The listing builds one solid part. Answer for the finished solid, in the listing's coordinates (mm). Face numbers are marked on the shaded views. A direction names the side the tool comes from. Round coordinates to 2 decimals unless told otherwise and drop trailing zeros. Write each loop counter-clockwise with the first axis right and the second up, starting at its lowest first coordinate (ties: lowest second). Pieces come first, ordered by that corner, then holes. Notation, with made-up numbers: (80.5, -29) - (112.5, -29) arc R11 cw to (112.5, -15) - close; hole circle Ø1 at (55.5, 72). An arc over 180 degrees is marked (long way). Use a Markdown table: item, result. Add a question column.
1) A cutting plane is placed at A-A (y = 11.25). Give the vertices of the cut face in (x, z) (3 decimals).
2) A cutting plane is placed at B-B (x = -10.5). Give the vertices of the cut face in (y, z), then the cut area to 3 significant figures.
3) A cutting plane is placed at D-D (z = 4.5). Give the vertices of the cut face in (x, y).
4) A tool of negligible diameter and unlimited length cuts with its end or side. For the marked faces 5, 6, 7 and 8, from which of +Z, -Z, +X, -X, +Y, -Y can it reach the whole face along a straight path? Write none if from no direction.
5) Determine the mould class of the marked faces 1, 2, 3 and 4 for opening direction X: +X half, -X half, draft (parallel to the pull), parting line (faces both ways), or undercut.
6) Each of these flat-tipped pins is pushed along its axis until it touches: P1, Ø2, axis at x = -22.5, z = -3.5, coming from the +Y side; P2, Ø0.6, axis at y = 2, z = 6, coming from the +X side; P3, Ø0.7, axis at y = 0.5, z = 5.5, coming from the +X side (3 decimals); P4, Ø3, axis at x = -5.5, z = 3.5, coming from the +Y side. Where does it stop, or does it pass through?
7) A cutting plane is placed at C-C (z = -4.5). Give the vertices of the cut face in (x, y) (3 decimals).
8) Find the intervals of material crossed by probe 1 along X at (y, z) = (1.1, 3.1) (3 decimals); probe 2 along X at (y, z) = (2.1, 3.1) (3 decimals); probe 3 along X at (y, z) = (9, -2.5) (3 decimals), in increasing order. Write a range as from..to.
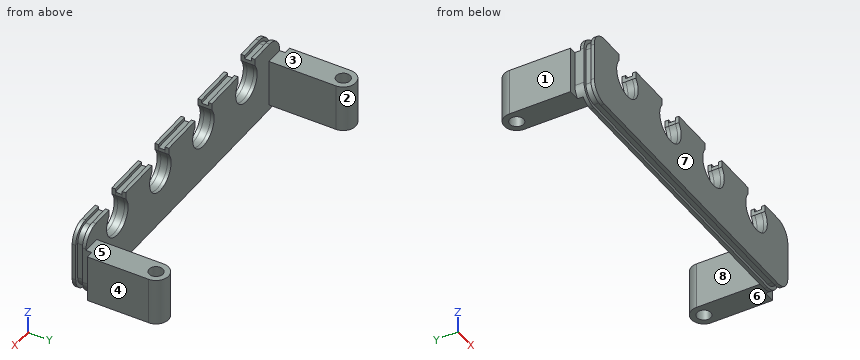
```python
from build123d import *
from build123d import SkipClean  # not in build123d's __all__

# Parameters (mm, degrees)
F1_DEPTH = 0.64
F3_DEPTH = 1.21
F5_DEPTH = 0.64
F7_R     = 1.25
F8_DEPTH = 8.5
F9_DEPTH = 1


# Not quite as in the source:
# - after a boolean that leaves OpenCascade's solid faulty, fix() repairs it


with BuildPart() as f1:
    # F0 (on Front) → F1 (new body)
    with BuildSketch(Plane.XZ):
        with BuildLine():
            ThreePointArc((-29.225, -3.35), (-28.3463203436, -5.4713203436), (-26.225, -6.35))
            Line((-26.225, -6.35), (26.225, -6.35))
            ThreePointArc((26.225, -6.35), (28.3463203436, -5.4713203436), (29.225, -3.35))
            Line((29.225, -3.35), (29.225, 3.35))
            ThreePointArc((29.225, 3.35), (28.3463203436, 5.4713203436), (26.225, 6.35))
            Line((26.225, 6.35), (22.325, 6.35))
            Line((22.325, 6.35), (22.325, 5.114944168))
            ThreePointArc((22.325, 5.114944168), (19.775, -0.15), (17.225, 5.114944168))
            Line((17.225, 5.114944168), (17.225, 6.35))
            Line((17.225, 6.35), (9.325, 6.35))
            Line((9.325, 6.35), (9.325, 5.114944168))
            ThreePointArc((9.325, 5.114944168), (6.775, -0.15), (4.225, 5.114944168))
            Line((4.225, 5.114944168), (4.225, 6.35))
            Line((4.225, 6.35), (-3.675, 6.35))
            Line((-3.675, 6.35), (-3.675, 5.114944168))
            ThreePointArc((-3.675, 5.114944168), (-6.225, -0.15), (-8.775, 5.114944168))
            Line((-8.775, 5.114944168), (-8.775, 6.35))
            Line((-8.775, 6.35), (-16.675, 6.35))
            Line((-16.675, 6.35), (-16.675, 5.114944168))
            ThreePointArc((-16.675, 5.114944168), (-19.225, -0.15), (-21.775, 5.114944168))
            Line((-21.775, 5.114944168), (-21.775, 6.35))
            Line((-21.775, 6.35), (-26.225, 6.35))
            ThreePointArc((-26.225, 6.35), (-28.3463203436, 5.4713203436), (-29.225, 3.35))
            Line((-29.225, 3.35), (-29.225, -3.35))
        make_face()
    extrude(amount=-F1_DEPTH)

    # F2 (on face) → F3 (join)
    with BuildSketch(Plane(origin=(0, 0.64, 0), x_dir=(-1, 0, 0), z_dir=(0, 1, 0))):
        with BuildLine():
            Line((-22.325, 5.114944168), (-22.325, 5.75))
            Line((-22.325, 5.75), (-26.225, 5.75))
            ThreePointArc((-26.225, 5.75), (-27.9220562748, 5.0470562748), (-28.625, 3.35))
            Line((-28.625, 3.35), (-28.625, -3.35))
            ThreePointArc((-28.625, -3.35), (-27.9220562748, -5.0470562748), (-26.225, -5.75))
            Line((-26.225, -5.75), (26.225, -5.75))
            ThreePointArc((26.225, -5.75), (27.9220562748, -5.0470562748), (28.625, -3.35))
            Line((28.625, -3.35), (28.625, 3.35))
            ThreePointArc((28.625, 3.35), (27.9220562748, 5.0470562748), (26.225, 5.75))
            Line((26.225, 5.75), (21.775, 5.75))
            Line((21.775, 5.75), (21.775, 5.114944168))
            ThreePointArc((21.775, 5.114944168), (19.225, -0.15), (16.675, 5.114944168))
            Line((16.675, 5.114944168), (16.675, 5.75))
            Line((16.675, 5.75), (8.775, 5.75))
            Line((8.775, 5.75), (8.775, 5.114944168))
            ThreePointArc((8.775, 5.114944168), (6.225, -0.15), (3.675, 5.114944168))
            Line((3.675, 5.114944168), (3.675, 5.75))
            Line((3.675, 5.75), (-4.225, 5.75))
            Line((-4.225, 5.75), (-4.225, 5.114944168))
            ThreePointArc((-4.225, 5.114944168), (-6.775, -0.15), (-9.325, 5.114944168))
            Line((-9.325, 5.114944168), (-9.325, 5.75))
            Line((-9.325, 5.75), (-17.225, 5.75))
            Line((-17.225, 5.75), (-17.225, 5.114944168))
            ThreePointArc((-17.225, 5.114944168), (-19.775, -0.15), (-22.325, 5.114944168))
        make_face()
    with SkipClean():  # cleaning this boolean's faces spoils the solid; the shape is the same uncleaned
        extrude(amount=F3_DEPTH)

    # F4 (on face) → F5 (join)
    with BuildSketch(Plane(origin=(0, 1.85, 0), x_dir=(-1, 0, 0), z_dir=(0, 1, 0))):
        with BuildLine():
            ThreePointArc((-29.225, -3.35), (-28.3463203436, -5.4713203436), (-26.225, -6.35))
            Line((-26.225, -6.35), (26.225, -6.35))
            ThreePointArc((26.225, -6.35), (28.3463203436, -5.4713203436), (29.225, -3.35))
            Line((29.225, -3.35), (29.225, 3.35))
            ThreePointArc((29.225, 3.35), (28.3463203436, 5.4713203436), (26.225, 6.35))
            Line((26.225, 6.35), (21.775, 6.35))
            Line((21.775, 6.35), (21.775, 5.114944168))
            ThreePointArc((21.775, 5.114944168), (19.225, -0.15), (16.675, 5.114944168))
            Line((16.675, 5.114944168), (16.675, 6.35))
            Line((16.675, 6.35), (8.775, 6.35))
            Line((8.775, 6.35), (8.775, 5.114944168))
            ThreePointArc((8.775, 5.114944168), (6.225, -0.15), (3.675, 5.114944168))
            Line((3.675, 5.114944168), (3.675, 6.35))
            Line((3.675, 6.35), (-4.225, 6.35))
            Line((-4.225, 6.35), (-4.225, 5.114944168))
            ThreePointArc((-4.225, 5.114944168), (-6.775, -0.15), (-9.325, 5.114944168))
            Line((-9.325, 5.114944168), (-9.325, 6.35))
            Line((-9.325, 6.35), (-17.225, 6.35))
            Line((-17.225, 6.35), (-17.225, 5.114944168))
            ThreePointArc((-17.225, 5.114944168), (-19.775, -0.15), (-22.325, 5.114944168))
            Line((-22.325, 5.114944168), (-22.325, 6.35))
            Line((-22.325, 6.35), (-26.225, 6.35))
            ThreePointArc((-26.225, 6.35), (-28.3463203436, 5.4713203436), (-29.225, 3.35))
            Line((-29.225, 3.35), (-29.225, -3.35))
        make_face()
    extrude(amount=F5_DEPTH)

    add(f1.part.fix(), mode=Mode.REPLACE)

    # F7 (on offset) → F8 (join)
    with BuildSketch(Plane(origin=(0, 0, -5.4), x_dir=(1, 0, 0), z_dir=(0, 0, -1))):
        with BuildLine():
            Line((29.225, -3.49), (29.225, -2.49))
            Line((29.225, -2.49), (26.025, -2.49))
            Line((26.025, -2.49), (26.025, -3.49))
            Line((26.025, -3.49), (26.025, -14.49))
            ThreePointArc((26.025, -14.49), (28.275, -16.74), (30.525, -14.49))
            Line((30.525, -14.49), (30.525, -3.49))
            Line((30.525, -3.49), (29.225, -3.49))
        make_face()
        with Locations((28.275, -14.49)):
            Circle(F7_R, mode=Mode.SUBTRACT)
        with BuildLine():
            Line((-26.025, -14.49), (-26.025, -3.49))
            Line((-26.025, -3.49), (-26.025, -2.49))
            Line((-26.025, -2.49), (-29.225, -2.49))
            Line((-29.225, -2.49), (-29.225, -3.49))
            Line((-29.225, -3.49), (-30.525, -3.49))
            Line((-30.525, -3.49), (-30.525, -14.49))
            ThreePointArc((-30.525, -14.49), (-28.275, -16.74), (-26.025, -14.49))
        make_face()
        with Locations((-28.275, -14.49)):
            Circle(F7_R, mode=Mode.SUBTRACT)
    extrude(amount=-F8_DEPTH)

    # F9 (cut): faces of the model
    f9_faces = [f1.faces().sort_by_distance(p)[0] for p in [
        (28.9889729085, 2.49, -4.9023634763),
        (-28.9889729085, 2.49, -4.9023634763),
    ]]
    extrude(f9_faces, amount=-F9_DEPTH, mode=Mode.SUBTRACT)


solid = f1.part
```
Entries:
| question | item | result |
|---|---|---|
| 1 | outline | (-30.525, -5.4) - (-26.025, -5.4) - (-26.025, 3.1) - (-30.525, 3.1) - close; (26.025, -5.4) - (30.525, -5.4) - (30.525, 3.1) - (26.025, 3.1) - close |
| 2 | outline | (0, -6.35) - (0.64, -6.35) - (0.64, -5.75) - (1.85, -5.75) - (1.85, -6.35) - (2.49, -6.35) - (2.49, 6.35) - (1.85, 6.35) - (1.85, 5.75) - (0.64, 5.75) - (0.64, 6.35) - (0, 6.35) - close |
| 2 | area | 30.2 mm² |
| 3 | outline | (-29, 0) - (-22.16, 0) - (-22.16, 2.49) - (-29, 2.49) - (-29, 1.85) - (-28.33, 1.85) - (-28.33, 0.64) - (-29, 0.64) - close; (-16.29, 0) - (-9.16, 0) - (-9.16, 2.49) - (-16.29, 2.49) - close; (-3.29, 0) - (3.84, 0) - (3.84, 2.49) - (-3.29, 2.49) - close; (9.71, 0) - (16.84, 0) - (16.84, 2.49) - (9.71, 2.49) - close; (22.71, 0) - (29, 0) - (29, 0.64) - (28.33, 0.64) - (28.33, 1.85) - (29, 1.85) - (29, 2.49) - (22.71, 2.49) - close |
| 4 | face 5 | +Z, +X, -X, +Y |
| 4 | face 6 | -Z, +X, -X, +Y |
| 4 | face 7 | +Z, -Z, +X, -X, -Y |
| 4 | face 8 | +Z, -Z, +Y |
| 5 | face 1 | -X half |
| 5 | face 2 | undercut |
| 5 | face 3 | draft |
| 5 | face 4 | +X half |
| 6 | P1 | stops at y = 2.49 |
| 6 | P2 | stops at x = 28.09 |
| 6 | P3 | stops at x = 28.625 |
| 6 | P4 | passes through |
| 7 | outline | (-30.525, 3.49) - (-28.996, 3.49) - (-28.996, 1.85) - (-28.332, 1.85) - (-28.332, 0.64) - (-28.996, 0.64) - (-28.996, 0) - (28.996, 0) - (28.996, 0.64) - (28.332, 0.64) - (28.332, 1.85) - (28.996, 1.85) - (28.996, 3.49) - (30.525, 3.49) - (30.525, 14.49) arc R2.25 ccw to (26.025, 14.49) - (26.025, 2.49) - (-26.025, 2.49) - (-26.025, 14.49) arc R2.25 ccw to (-30.525, 14.49) - close; hole circle Ø2.5 at (-28.275, 14.49); hole circle Ø2.5 at (28.275, 14.49) |
| 8 | probe 1 | x = -28.625..-22.475, -15.975..-9.475, -2.975..3.525, 10.025..16.525, 23.025..28.625 |
| 8 | probe 2 | x = -29.225..-22.475, -15.975..-9.475, -2.975..3.525, 10.025..16.525, 23.025..29.225 |
| 8 | probe 3 | x = -30.525..-26.025, 26.025..30.525 |
